```python
from build123d import *

# Parameters (mm, degrees)
ESQUISSE2_R             = 2.5
ENL_V_MAT_EXTRU_1_DEPTH = 48.72970773


with BuildPart() as part:
    # Esquisse1 → Révolution1 (revolve)
    with BuildSketch(Plane.XY, mode=Mode.PRIVATE) as r_volution1_sk:
        Polygon((4, 0), (28.75, 0), (28.75, 4.5), (12, 4.5), (12, 25), (4, 25), align=None)
    revolve(r_volution1_sk.sketch.rotate(Axis((0, 0, 0), (0, 1, 0)), 90), axis=Axis((0, 0, 0), (0, 1, 0)))

    # Esquisse2 → Enlèv. mat.-Extru.1 (cut, through all)
    with BuildSketch(Plane.XZ):
        with Locations(Location((23.75, 0, 0), (0, 0, 270))):
            Circle(ESQUISSE2_R)
        with Locations(Location((11.875, -20.56810334, 0), (0, 0, 270))):
            Circle(ESQUISSE2_R)
        with Locations(Location((-11.875, -20.56810334, 0), (0, 0, 270))):
            Circle(ESQUISSE2_R)
        with Locations(Location((-23.75, 0, 0), (0, 0, 270))):
            Circle(ESQUISSE2_R)
        with Locations(Location((-11.875, 20.56810334, 0), (0, 0, 270))):
            Circle(ESQUISSE2_R)
        with Locations(Location((11.875, 20.56810334, 0), (0, 0, 270))):
            Circle(ESQUISSE2_R)
    extrude(amount=-ENL_V_MAT_EXTRU_1_DEPTH, mode=Mode.SUBTRACT)


solid = part.part
```
Work out the finished part from the listing and answer in its coordinate system (mm). A direction names the side the tool comes from. Give positions to 0.01 mm unless a question says otherwise; leave off trailing zeros. Loops run counter-clockwise (first coordinate to the right, second up) from the corner with the lowest first, then second, coordinate; pieces in that order, holes last. Notation, with made-up numbers: (-26, 83.5) -> (-22, 83.5) arc R32 ccw to (-22, 120.5) -> close; hole circle Ø8 at (83.25, 88). An arc over 180 degrees is marked (long way). Put each result on its own line as item: value. Start each with the question number.
Item 1: Find the intervals of material crossed by L1, parallel to X at y = 2.5, z = 0; L2, parallel to Y at x = 9.5, z = -14; L3, parallel to Z at x = 7, y = 12.5, in increasing order. Write a range as [from, to].
Item 2: The part is cut by section D-D (z = 7.5). Give the vertices of the cut face in (x, y).
Item 3: The part is cut by section B-B (z = 0). Give the vertices of the cut face in (x, y), then the cut area to 3 significant figures.
Item 4: Each of these flat-tipped pins is pushed along its axis until it touches: P1, Ø2, axis at x = 1.5, y = 19.5, coming from the +Z side; P2, Ø8, axis at x = -23.75, z = 0, coming from the +Y side; P3, Ø4, axis at x = -15, y = 20.5, coming from the +Z side; P4, Ø10, axis at x = -0.5, z = 10.5, coming from the -Y side. Where does it stop, or does it pass through?
Item 5: Which of the six approach directions +Z, -Z, +X, -X, +Y, -Y give full straight-line access (tool end or side, diameter ignored) to faces 1 (the face through (26.23, 2.22, 0.33)), 2 (the face through (-0.4, 4.5, -12.4))?
Item 6: The mould has two halves that part along Z. Classify faces 3 (the face through (-3.604, 14.894, -11.446)), 4 (the face through (0, 0, 6)), 5 (the face through (9.657, 2.218, -21.722)): released by +Z, released by -Z, zero draft, split by the parting line, or undercut.
Item 7: The part is cut by section C-C (y = 5.75). Give the vertices of the cut face in (x, z), then the cut area to 3 significant figures.
Item 8: The part is cut by section A-A (x = -23.75). Give the vertices of the cut face in (y, z), then the cut area to 3 significant figures.
Answers below:
1. L1: [-28.75, -26.25], [-21.25, -4], [4, 21.25], [26.25, 28.75]
1. L2: [0, 4.5]
1. L3: [-9.75, 9.75]
2. outline: (-27.75, 0) -> (27.75, 0) -> (27.75, 4.5) -> (9.37, 4.5) -> (9.37, 25) -> (-9.37, 25) -> (-9.37, 4.5) -> (-27.75, 4.5) -> close
3. outline: (-28.75, 0) -> (-26.25, 0) -> (-26.25, 4.5) -> (-28.75, 4.5) -> close; (-21.25, 0) -> (-4, 0) -> (-4, 25) -> (-12, 25) -> (-12, 4.5) -> (-21.25, 4.5) -> close; (4, 0) -> (21.25, 0) -> (21.25, 4.5) -> (12, 4.5) -> (12, 25) -> (4, 25) -> close; (26.25, 0) -> (28.75, 0) -> (28.75, 4.5) -> (26.25, 4.5) -> close
3. area: 506 mm2
4. P1: z = 11.99
4. P2: y = 4.5
4. P3: through
4. P4: y = 0
5. face 1: +Y, -Y
5. face 2: +Y
6. face 3: split by the parting line
6. face 4: zero draft
6. face 5: undercut
7. outline: circle Ø24 at (0, 0); hole circle Ø8 at (0, 0)
7. area: 402 mm2
8. outline: (0, -16.2) -> (4.5, -16.2) -> (4.5, -2.5) -> (0, -2.5) -> close; (0, 2.5) -> (4.5, 2.5) -> (4.5, 16.2) -> (0, 16.2) -> close
8. area: 123 mm2
